from build123d import *

# Parameters (mm, degrees)
F1_DEPTH = 254
F2_R     = 215.9
F3_DEPTH = 12.7
F5_DEPTH = 381.001
F6_R     = 25.4


with BuildPart() as f1:
    # F0 (on Front) → F1 (new body)
    with BuildSketch(Plane.XZ):
        Polygon((-152.4, 12.7), (-152.4, 457.2), (-165.1, 457.2), (-165.1, 0), (165.1, 0), (165.1, 457.2), (152.4, 457.2), (152.4, 12.7), align=None)
    extrude(amount=F1_DEPTH)

    # F2 (on face) → F3 (join)
    with BuildSketch(Plane(origin=(0, 0, 0), x_dir=(1, 0, 0), z_dir=(0, 0, -1))):
        with Locations((0, 127)):
            Circle(F2_R)
    extrude(amount=F3_DEPTH)

    # F4 (on face) → F5 (cut, through all)
    with BuildSketch(Plane.YZ.offset(165.1)):
        with BuildLine():
            Line((-50.8, 457.2), (-203.2, 457.2))
            ThreePointArc((-203.2, 457.2), (-127, 381), (-50.8, 457.2))
        make_face()
    extrude(amount=-F5_DEPTH, mode=Mode.SUBTRACT)

    # F6
    f6_edges = [f1.edges().sort_by_distance(p)[0] for p in [
        (158.75, -254, 457.2),
        (158.75, 0, 457.2),
        (-158.75, 0, 457.2),
        (-158.75, -254, 457.2),
    ]]
    fillet(f6_edges, radius=F6_R)


solid = f1.part
Work out the finished part from the listing and answer in its coordinate system (mm). A direction names the side the tool comes from. Coordinates: 2 decimals unless noted, no trailing zeros. Loops run counter-clockwise (first coordinate to the right, second up) from the corner with the lowest first, then second, coordinate; pieces in that order, holes last. Notation, with made-up numbers: (15.5, 33) -> (45.5, 33) arc R21 cw to (45.5, 58) -> close; hole circle Ø8 at (37.25, 76.25). An arc over 180 degrees is marked (long way). Write each question's results on one line, items separated by ' | '. Start each with the question number.
1) Flat-ended cylindrical pins translate along their axes: P1, Ø10, axis at x = 30.5, y = 14.5, coming from the +Z side; P2, Ø4, axis at x = 88, y = -228.5, coming from the +Z side; P3, Ø6, axis at y = -58.5, z = 138.5, coming from the +X side. Find the tip coordinate at first contact, or state that the pin passes through.
2) Find section D-D on x = 104.5. Determine the outline of the cut face in (y, z).
3) For faces 1 (the flat face through (-1, -254, 9)), 2 (the flat face through (-165.1, -125, 232)), 3 (the flat face through (152.4, -125, 238)), determine the directions among +Z, -Z, +X, -X, +Y, -Y from which every point of the face is accessible in a straight line to the end or side of a thin tool.
4) The mould has two halves that part along X. Classify faces 4 (the flat face through (-3, -130, -12.7)), 5 (the flat face through (-152.4, -125, 232)), 6 (the flat face through (165.1, -125, 225)): pulls with the +X half, pulls with the -X half, needs draft (parallel to the pull), parting line crosses it, or undercut.
5) Find section A-A on z = 204.5. Determine the outline of the cut face in (x, y), then the cut area to 3 significant figures.
6) Find section B-B on y = -127. Determine the outline of the cut face in (x, z), then the cut area to 3 significant figures.
7) Consider line 1 along X through (y, z) = (-152.5, 28); line 2 along Z through (x, y) = (27, 44); line 3 along Z through (x, y) = (-48, -241.5). Determine where each line is inside the solid, lowest interval first.
8) Find section C-C on x = 0. Determine the outline of the cut face in (y, z), then the cut area to 3 significant figures.
Response values:
1) P1: stops at z = 0 | P2: stops at z = 12.7 | P3: stops at x = 165.1
2) outline: (-315.92, -12.7) -> (61.92, -12.7) -> (61.92, 0) -> (0, 0) -> (0, 12.7) -> (-254, 12.7) -> (-254, 0) -> (-315.92, 0) -> close
3) face 1: +Z, +X, -X, -Y | face 2: +Z, -X, +Y, -Y | face 3: +Z, +Y, -Y
4) face 4: needs draft | face 5: undercut | face 6: pulls with the +X half
5) outline: (-165.1, -254) -> (-152.4, -254) -> (-152.4, 0) -> (-165.1, 0) -> close; (152.4, -254) -> (165.1, -254) -> (165.1, 0) -> (152.4, 0) -> close | area: 6,450 mm^2
6) outline: (-215.9, -12.7) -> (215.9, -12.7) -> (215.9, 0) -> (165.1, 0) -> (165.1, 381) -> (152.4, 381) -> (152.4, 12.7) -> (-152.4, 12.7) -> (-152.4, 381) -> (-165.1, 381) -> (-165.1, 0) -> (-215.9, 0) -> close | area: 19,000 mm^2
7) line 1: x = -165.1 to -152.4, 152.4 to 165.1 | line 2: z = -12.7 to 0 | line 3: z = -12.7 to 12.7
8) outline: (-342.9, -12.7) -> (88.9, -12.7) -> (88.9, 0) -> (0, 0) -> (0, 12.7) -> (-254, 12.7) -> (-254, 0) -> (-342.9, 0) -> close | area: 8,710 mm^2
